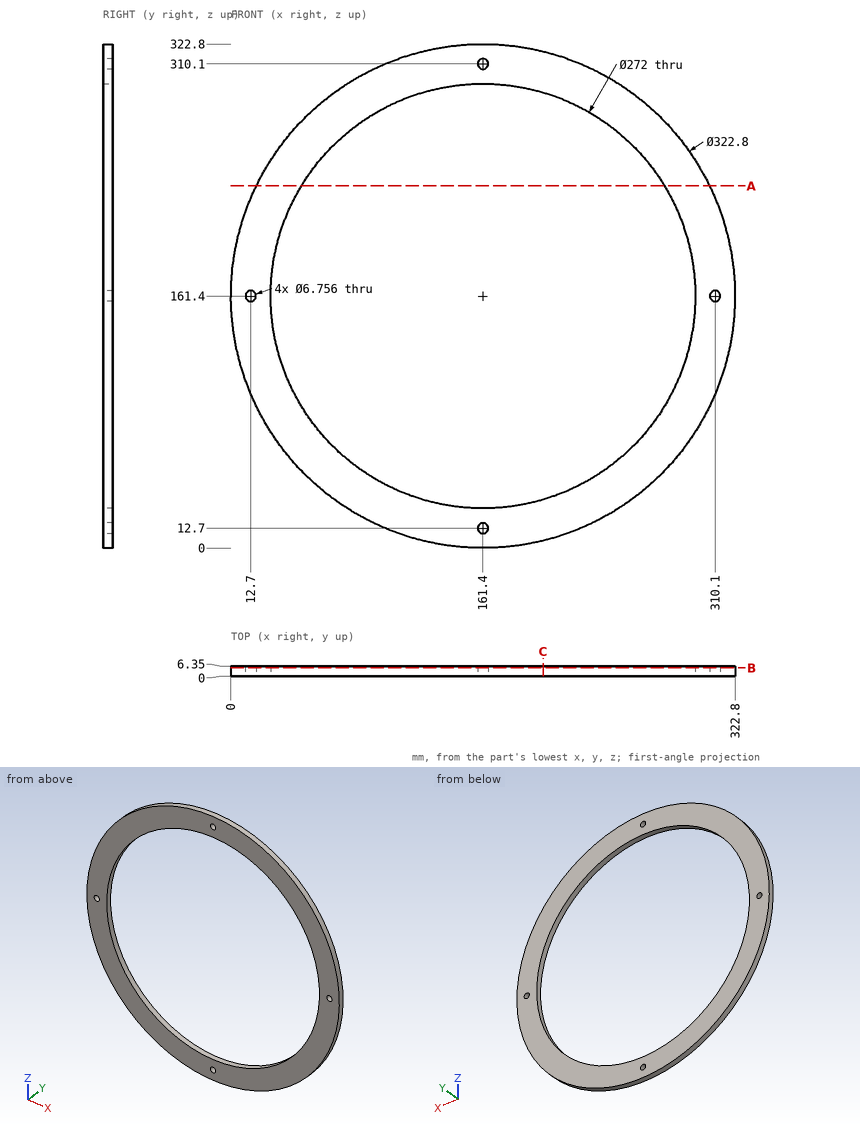
Design review of the part shown in the three views and the two pictorial views. Dimensions are in mm from the part's minimum x, y and z. Round coordinates to 2 decimals unless told otherwise and drop trailing zeros. Order: outer loops, then holes, each group sorted by start corner. A loop starts at its lowest first (then second) coordinate and runs counter-clockwise, first axis right, second up.
(1) For P1, Ø1.5, axis at y = 3, z = 129, coming from the -X side; P2, Ø1.5, axis at x = 198, y = 1, coming from the +Z side; P3, Ø11, axis at x = 310.1, z = 161.4, coming from the +Y side; P4, Ø3, axis at y = 3, z = 240.5, coming from the +X side, all flat-tipped, find the tip position at first contact; note any pin that passes through.
Working result:
P1: stops at x = 3.13
P2: stops at z = 318.77
P3: stops at y = 6.35
P4: stops at x = 302.92
(2) Take a section at B-B, the plane y = 5.25. State the section outline as (x, z) points.
Working result:
outline: circle Ø322.8 at (161.4, 161.4); hole circle Ø6.76 at (12.7, 161.4); hole circle Ø272 at (161.4, 161.4); hole circle Ø6.76 at (161.4, 12.7); hole circle Ø6.76 at (161.4, 310.1); hole circle Ø6.76 at (310.1, 161.4)
(3) Wall thickness on L1, parallel to X at y = 4.5, z = 161.4; L2, parallel to Z at x = 40, y = 1 (1 decimal); L3, parallel to X at y = 1.75, z = 126: over which ranges is each line inside the solid? List them lowest first.
Working result:
L1: x = 0 to 9.32, 16.08 to 25.4, 297.4 to 306.72, 313.48 to 322.8
L2: z = 55 to 100.1, 222.7 to 267.8
L3: x = 3.93 to 30.09, 292.71 to 318.87
(4) Take a section at A-A, the plane z = 232. State the section outline as (x, y) points, plus the area to 3 significant figures.
Working result:
outline: (16.26, 0) - (45.16, 0) - (45.16, 6.35) - (16.26, 6.35) - close; (277.64, 0) - (306.54, 0) - (306.54, 6.35) - (277.64, 6.35) - close
area: 367 mm2
(5) Take a section at C-C, the plane x = 200. State the section outline as (y, z) points.
Working result:
outline: (0, 4.68) - (6.35, 4.68) - (6.35, 30.99) - (0, 30.99) - close; (0, 291.81) - (6.35, 291.81) - (6.35, 318.12) - (0, 318.12) - close
